Here's how the part is built. I have some questions about the finished solid (model axes, mm). Face numbers are marked on the shaded views. Coordinates: 2 decimals unless noted, no trailing zeros. Write each loop counter-clockwise with the first axis right and the second up, starting at its lowest first coordinate (ties: lowest second). Pieces come first, ordered by that corner, then holes.
(1) Imagine slicing it at A-A, the plane x = 0. List the corners of the cut face in (y, z) for me, plus the area to 3 significant figures.
(2) Imagine slicing it at D-D, the plane z = 0.5. List the corners of the cut face in (x, y) for me, plus the area to 3 significant figures.
(3) For pin 1 Ø1.5 at (y, z) = (7.5, 1) entering from +X; pin 2 Ø4 at (y, z) = (5.5, 0) entering from -X; pin 3 Ø4.5 at (x, y) = (0, 0) entering from +Z, each with a flat end and sliding along its axis, tell me the tip position at first contact or that it passes through.
(4) Thinking about a two-plate mould opening in Y: for the marked faces 1, 2 and 3, which applies, released by +Y, released by -Y, zero draft, split by the parting line, or undercut?
(5) Please list where these lines run through material, in increasing order: probe 1 along Y at (x, z) = (0, 0.15); probe 2 along Z at (x, y) = (-2, 5.5); probe 3 along Y at (x, z) = (-1.75, 2).
(6) Imagine slicing it at B-B, the plane z = -2. List the corners of the cut face in (x, y) for me, plus the area to 3 significant figures.
(7) Imagine slicing it at C-C, the plane y = 9.75. List the corners of the cut face in (x, z) for me, plus the area to 3 significant figures.
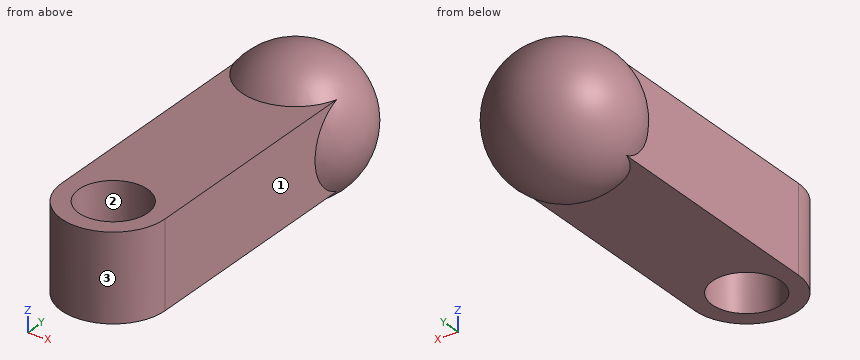
```python
from build123d import *

# Parameters (mm, degrees)
SALIENTE_EXTRUIR1_DEPTH      = 2.5
SALIENTE_EXTRUIR1_DEPTH_BACK = 2.5
CROQUIS1_R                   = 2


with BuildPart() as part:
    # Croquis1 → Saliente-Extruir1 (new, two sides: drawn at the far end of the back side and taken through both)
    with BuildSketch(Plane.XY.offset(-SALIENTE_EXTRUIR1_DEPTH_BACK)):
        with BuildLine():
            Line((3, 15), (3, 0))
            ThreePointArc((3, 0), (0, -3), (-3, 0))
            Line((-3, 0), (-3, 15))
            ThreePointArc((-3, 15), (0, 18), (3, 15))
        make_face()
        Circle(CROQUIS1_R, mode=Mode.SUBTRACT)
        with Locations((0, 15)):
            Circle(CROQUIS1_R, mode=Mode.SUBTRACT)
    extrude(amount=SALIENTE_EXTRUIR1_DEPTH + SALIENTE_EXTRUIR1_DEPTH_BACK)

    # Croquis2 → Revolución1 (revolve)
    with BuildSketch(Plane.XY):
        with BuildLine():
            Line((0, 11), (0, 19))
            ThreePointArc((0, 19), (4, 15), (0, 11))
        make_face()
    revolve(axis=Axis((0, 11, 0), (0, 1, 0)))


solid = part.part
```
Recorded:
1. outline: (-3, -2.5) - (-2, -2.5) - (-2, 2.5) - (-3, 2.5) - close; (2, -2.5) - (11.88, -2.5) arc R4 ccw (long way) to (11.88, 2.5) - (2, 2.5) - close
1. area: 102 mm2
2. outline: (-3, 0) arc R3 ccw to (3, 0) - (3, 12.4) arc R3.97 ccw (long way) to (-3, 12.4) - close; hole circle Ø4 at (0, 0)
2. area: 120 mm2
3. pin 1: stops at x = 3
3. pin 2: stops at x = -3
3. pin 3: stops at z = 2.5
4. face 1: zero draft
4. face 2: undercut
4. face 3: released by -Y
5. probe 1: y = -3 to -2, 2 to 19
5. probe 2: z = -2.5 to 2.5
5. probe 3: y = -2.44 to -0.97, 0.97 to 17.99
6. outline: (-3, 0) arc R3 ccw to (3, 0) - (3, 13.27) arc R3.46 ccw (long way) to (-3, 13.27) - close; hole circle Ø4 at (0, 0)
6. area: 112 mm2
7. outline: (-3, -2.5) - (3, -2.5) - (3, 2.5) - (-3, 2.5) - close
7. area: 30.0 mm2
